Geometry check sheet. Reference: the model listing, model coordinates, mm. A direction names the side the tool comes from. Round coordinates to 2 decimals unless told otherwise and drop trailing zeros. Order: outer loops, then holes, each group sorted by start corner. A loop starts at its lowest first (then second) coordinate and runs counter-clockwise, first axis right, second up. Notation, with made-up numbers: (-14.5, 66.25) - (17.5, 66.25) arc R21 ccw to (17.5, 70.25) - close; hole circle Ø10 at (37.5, 51.25). An arc over 180 degrees is marked (long way). Write each question's results on one line, items separated by ' | '.
```python
from build123d import *

# Parameters (mm, degrees)
F0_R          = 1
F1_DEPTH      = 6
F1_DEPTH_BACK = 6
F2_R          = 1
F3_W          = 6
F3_H          = 4
F4_DEPTH      = 4
F5_R          = 2
F5_R_2        = 1
F6_DEPTH      = 1
F7_W          = 4
F7_H          = 6
F8_DEPTH      = 2
F9_R          = 1
F10_DEPTH     = 3


with BuildPart() as f1:
    # F0 (on Front) → F1 (new body, two sides)
    with BuildSketch(Plane.XZ) as f1_sk:
        Polygon((0, 6), (0, 0), (4, 0), (4, 6), (4, 10), (0, 10), (-4, 10), (-4, 6), align=None)
        with Locations((-2, 8)):
            Circle(F0_R, mode=Mode.SUBTRACT)
    extrude(amount=F1_DEPTH)
    extrude(f1_sk.sketch, amount=-F1_DEPTH_BACK)

    # F2
    f2_edges = [f1.edges().sort_by_distance(p)[0] for p in [
        (-4, 0, 10),
        (-4, 0, 6),
    ]]
    fillet(f2_edges, radius=F2_R)

    # F3 (on face) → F4 (cut, through all)
    with BuildSketch(Plane(origin=(-4, 0, 0), x_dir=(0, -1, 0), z_dir=(-1, 0, 0))):
        with Locations((0, 8)):
            Rectangle(F3_W, F3_H)
    extrude(amount=-F4_DEPTH, mode=Mode.SUBTRACT)

    # F5 (on face) → F6 (cut)
    with BuildSketch(Plane(origin=(0, 0, 0), x_dir=(0, -1, 0), z_dir=(-1, 0, 0))):
        with Locations((0, 2.5)):
            Circle(F5_R)
        with Locations((0, 2.5)):
            Circle(F5_R_2, mode=Mode.SUBTRACT)
    extrude(amount=-F6_DEPTH, mode=Mode.SUBTRACT)

    # F7 (on face) → F8 (join)
    with BuildSketch(Plane.XY.offset(10)):
        with Locations((2, 0)):
            Rectangle(F7_W, F7_H)
    extrude(amount=F8_DEPTH)

    # F9 (on face) → F10 (cut)
    with BuildSketch(Plane(origin=(0, 0, 0), x_dir=(0, -1, 0), z_dir=(-1, 0, 0))):
        with Locations((0, 10.5)):
            Circle(F9_R)
    extrude(amount=-F10_DEPTH, mode=Mode.SUBTRACT)


solid = f1.part
```
(1) Access from +Z, -Z, +X, -X, +Y, -Y to the whole of each face (thin tool, end or side, straight path). Record for faces 1 (the face through (-2, 4, 6)), 2 (the face through (1, -0.9, 1.6)), 3 (the face through (1, 4, 10)).
Answers follow:
face 1: -Z, -X, +Y, -Y | face 2: -X | face 3: +Z, +X, -X, +Y
(2) Section check C-C (x = -2). Record the cut outline in (y, z), then the cut area to 3 significant figures.
Answers follow:
outline: (-6, 6) - (-3, 6) - (-3, 7) - (-6, 7) - close; (-6, 9) - (-3, 9) - (-3, 10) - (-6, 10) - close; (3, 6) - (6, 6) - (6, 7) - (3, 7) - close; (3, 9) - (6, 9) - (6, 10) - (3, 10) - close | area: 12.0 mm²
(3) Section check A-A (x = 0.5). Record the cut outline in (y, z), then the cut area to 3 significant figures.
Answers follow:
outline: (-6, 0) - (6, 0) - (6, 10) - (3, 10) - (3, 12) - (-3, 12) - (-3, 10) - (-6, 10) - close; circle Ø2 at (0, 2.5); hole circle Ø4 at (0, 2.5); hole circle Ø2 at (0, 10.5) | area: 119 mm²
(4) Depth check by flat-ended pin: pin 1 Ø5 at (y, z) = (-4.5, 1.5) entering from -X; pin 2 Ø1.6 at (x, z) = (-2, 8) entering from -Y; pin 3 Ø0.9 at (x, y) = (1.5, -4) entering from +Z; pin 4 Ø1.5 at (x, y) = (-2.5, -4.5) entering from -Z. Enter the tip coordinate at first touch or a pass-through.
Answers follow:
pin 1: x = 0 | pin 2: through | pin 3: z = 10 | pin 4: z = 6
(5) Material ranges on line 1 (Z direction, x = 0.6, y = 0); line 2 (Z direction, x = -2, y = 5.4); line 3 (X direction, y = -4.05, z = 8), recorded low to high.
Answers follow:
line 1: 0 to 0.5, 1.5 to 3.5, 4.5 to 9.5, 11.5 to 12 | line 2: 6 to 7, 9 to 10 | line 3: -4 to -3, -1 to 4
(6) Draft check along Y on faces 4 (the face through (-2, 4, 9)), 5 (the face through (1, -6, 6)), 6 (the face through (-1, 3, 7)). Enter one of: released by +Y, released by -Y, zero draft, split by the parting line, or undercut.
Answers follow:
face 4: zero draft | face 5: released by -Y | face 6: undercut
(7) Section check B-B (z = 8). Record the cut outline in (x, y), then the cut area to 3 significant figures.
Answers follow:
outline: (-4, -6) - (-3, -6) - (-3, -3) - (-4, -3) - close; (-4, 3) - (-3, 3) - (-3, 6) - (-4, 6) - close; (-1, -6) - (4, -6) - (4, 6) - (-1, 6) - (-1, 3) - (0, 3) - (0, -3) - (-1, -3) - close | area: 60.0 mm²
(8) Section check D-D (x = -0.5). Record the cut outline in (y, z), then the cut area to 3 significant figures.
Answers follow:
outline: (-6, 6) - (-3, 6) - (-3, 10) - (-6, 10) - close; (3, 6) - (6, 6) - (6, 10) - (3, 10) - close | area: 24.0 mm²
